Could you check a few things on this model? Use its own coordinates, in mm. A direction names the side the tool comes from. Round coordinates to 2 decimals unless told otherwise and drop trailing zeros. Loops run counter-clockwise (first coordinate to the right, second up) from the corner with the lowest first, then second, coordinate; pieces in that order, holes last.
from build123d import *

# Parameters (mm, degrees)
SKETCH1_W           = 32
SKETCH1_H           = 32
BOSS_EXTRUDE1_DEPTH = 10
SKETCH2_W           = 32
SKETCH2_H           = 45
BOSS_EXTRUDE2_DEPTH = 41
SKETCH3_R           = 1.6
SKETCH3_R_2         = 6.5
CUT_EXTRUDE1_DEPTH  = 10


with BuildPart() as part:
    # Sketch1 → Boss-Extrude1 (new body)
    with BuildSketch(Plane.XY):
        Rectangle(SKETCH1_W, SKETCH1_H)
    extrude(amount=BOSS_EXTRUDE1_DEPTH)

    # Sketch2 → Boss-Extrude2 (add)
    with BuildSketch(Plane.XY.offset(10)):
        with Locations((0, 6.5)):
            Rectangle(SKETCH2_W, SKETCH2_H)
    extrude(amount=BOSS_EXTRUDE2_DEPTH)

    # Sketch3 → Cut-Extrude1 (cut)
    with BuildSketch(Plane(origin=(0, 0, 0), x_dir=(-1, 0, 0), z_dir=(0, 0, -1))):
        with Locations((-12, 12)):
            Circle(SKETCH3_R)
        with Locations((-12, -12)):
            Circle(SKETCH3_R)
        with Locations((12, 12)):
            Circle(SKETCH3_R)
        with Locations((12, -12)):
            Circle(SKETCH3_R)
        Circle(SKETCH3_R_2)
    extrude(amount=-CUT_EXTRUDE1_DEPTH, mode=Mode.SUBTRACT)


solid = part.part
Item 1: If we section it at C-C, the plane y = 12: Please give me the cut outline in (x, z), then the cut area to 3 significant figures.
Results list:
outline: (-16, 0) - (-13.6, 0) - (-13.6, 10) - (-10.4, 10) - (-10.4, 0) - (10.4, 0) - (10.4, 10) - (13.6, 10) - (13.6, 0) - (16, 0) - (16, 51) - (-16, 51) - close
area: 1,570 mm2
Item 2: If we section it at A-A, the plane y = 0: Please give me the cut outline in (x, z).
Results list:
outline: (-16, 0) - (-6.5, 0) - (-6.5, 10) - (6.5, 10) - (6.5, 0) - (16, 0) - (16, 51) - (-16, 51) - close
Item 3: Will this pin go through, and if not, where does the flat tip stop? pin 1 (10.5 mm diameter, centred on x = 0.5, y = 0, fed in from -Z).
Results list:
pin 1: stops at z = 10
Item 4: If we section it at D-D, the plane x = 4: Please give me the cut outline in (y, z), then the cut area to 3 significant figures.
Results list:
outline: (-16, 0) - (-5.12, 0) - (-5.12, 10) - (5.12, 10) - (5.12, 0) - (16, 0) - (16, 10) - (29, 10) - (29, 51) - (-16, 51) - close
area: 2,060 mm2
Item 5: If we section it at B-B, the plane x = 12: Please give me the cut outline in (y, z), then the cut area to 3 significant figures.
Results list:
outline: (-16, 0) - (-13.6, 0) - (-13.6, 10) - (-10.4, 10) - (-10.4, 0) - (10.4, 0) - (10.4, 10) - (13.6, 10) - (13.6, 0) - (16, 0) - (16, 10) - (29, 10) - (29, 51) - (-16, 51) - close
area: 2,100 mm2
Item 6: We'd pull the mould along Y, two halves only. Please class faces 1 (the flat face through (0, 7, 51)), 2 (the flat face through (0, 29, 30)), 3 (the flat face through (12, 12, 10)): released by +Y, released by -Y, zero draft, split by the parting line, or undercut.
Results list:
face 1: zero draft
face 2: released by +Y
face 3: undercut
Item 7: If I drill on line 1 along Y through (x, z) = (-12, 5.25); line 2 along Y through (x, z) = (0, 2); line 3 along Z through (x, y) = (4, 19), over which ranges is the centre line in solid material (lowest first)?
Results list:
line 1: y = -16 to -13.6, -10.4 to 10.4, 13.6 to 16
line 2: y = -16 to -6.5, 6.5 to 16
line 3: z = 10 to 51
Item 8: For faces 4 (the flat face through (0, 16, 5)), 5 (the flat face through (0, -16, 25)), 6 (the cylindrical face through (-10.4, -11.93, 4.93)), which set-ups out of +Z, -Z, +X, -X, +Y, -Y let a thin tool reach every point of the face, with its end or its side?
Results list:
face 4: -Z, +X, -X, +Y
face 5: +Z, -Z, +X, -X, -Y
face 6: -Z
